Geometry: final body of the model. Coordinates: model frame, mm. Coordinates: 2 decimals unless noted, no trailing zeros. Order: outer loops, then holes, each group sorted by start corner. A loop starts at its lowest first (then second) coordinate and runs counter-clockwise, first axis right, second up. Notation, with made-up numbers: M 27.25,82 L 71.25,82 A17 ccw 71.25,93 Z; hole C 58,64 d8. An arc over 180 degrees is marked long. One line per question, with ' | ' between items.
Autodesk Inventor part; units mm, degrees
ref_plane "YZ Plane" through (0, 0, 0) normal (1, 0, 0) x (0, 1, 0)
ref_plane "XZ Plane" through (0, 0, 0) normal (0, 1, 0) x (-1, 0, 0)
ref_plane "XY Plane" through (0, 0, 0) normal (0, 0, 1) x (1, 0, 0)
sketch "スケッチ1" plane through (0, 0, 0) normal (0, 0, 1) x (1, 0, 0)
  line L0 (51.397, 0) -> (6, 70) construction
  line L1 (51.397, 0) -> (65, -20.9752)
  line L2 (65, -20.9752) -> (25, -44.6993)
  line L3 (0, 0) -> (0, 56.1205) construction
  line L4 (0, 0) -> (51.397, 0) construction
  arc A0 (17.9848, 26.067) -> (17.1698, 21.0636) centre (51.7641, 17.9963) ccw construction
  arc A1 (10.2038, 27.926) -> (9.201, 21.7701) centre (51.7641, 17.9963) ccw construction
  arc A2 (9.201, 21.7701) -> (17.1698, 21.0636) centre (13.1854, 21.4169) ccw construction
  line L5 (13.1854, 21.4169) -> (51.7641, 17.9963) construction
  line L6 (51.7641, 17.9963) -> (13.5604, 24.3596)
  arc A3 (13.5604, 24.3596) -> (13.1854, 21.4169) centre (51.7641, 17.9963) ccw construction
  line L7 (13.1854, 21.4169) -> (66.7927, -23.5971) construction
  line L8 (66.7927, -23.5971) -> (61.9625, 22.6577) construction
  line L9 (13.5604, 24.3596) -> (25, -44.6993)
  line L10 (13.5604, 24.3596) -> (6, 70) construction
  line L11 (13.5604, 24.3596) -> (51.397, 0) construction
  arc A4 (51.397, -25) -> (61.9625, 22.6577) centre (51.397, 0) ccw
  line L12 (25, -44.6993) -> (65, -44.6993) construction
  line L13 (65, -44.6993) -> (65, -20.9752) construction
  line L14 (45, -44.6993) -> (45, -284.6993) construction
  line L15 (51.397, 0) -> (51.9579, -2.4363)
  line L16 (51.397, 0) -> (50.5419, -2.3492) construction
  arc A5 (50.5419, -2.3492) -> (53.1648, 1.7678) centre (51.397, 0) ccw construction
  line L17 (51.397, 0) -> (51.3697, -2.4999) construction
  line L18 (51.397, 0) -> (52.2006, -2.3673) construction
  line L19 (51.397, 0) -> (52.9404, -1.9667) construction
  line L20 (51.397, 0) -> (53.5055, -1.3432) construction
  line L21 (51.397, 0) -> (53.8317, -0.5677) construction
  line L22 (51.397, 0) -> (53.8821, 0.2722) construction
  line L23 (51.397, 0) -> (53.6511, 1.0812) construction
  line L24 (51.397, 0) -> (53.1648, 1.7678) construction
  line L25 (51.7641, 17.9963) -> (51.9579, -2.4363)
  line L26 (50.5419, -2.3492) -> (51.7641, 17.9963) construction
  line L27 (51.7641, 17.9963) -> (53.1648, 1.7678) construction
  line L28 (51.397, -8) -> (51.397, -25) construction
  line L29 (54.051, -7.5469) -> (59.6907, -23.5842) construction
  line L30 (56.4044, -6.2391) -> (67.0451, -19.4971) construction
  line L31 (58.1906, -4.2245) -> (72.6271, -13.2017) construction
  line L32 (59.2074, -1.7315) -> (75.8044, -5.411) construction
  line L33 (59.3395, 0.9576) -> (76.2172, 2.9926) construction
  line L34 (58.572, 3.5383) -> (73.8188, 11.0572) construction
  line L35 (56.9918, 5.7182) -> (68.8808, 17.8694) construction
  line L36 (54.7779, 7.2505) -> (61.9625, 22.6577) construction
  arc A6 (51.397, -8) -> (54.7779, 7.2505) centre (51.397, 0) ccw construction
  line L37 (14.0943, 26.9965) -> (51.7641, 17.9963) construction
  arc A7 (14.0943, 26.9965) -> (13.5604, 24.3596) centre (51.7641, 17.9963) ccw construction
  arc A8 (17.9848, 26.067) -> (10.2038, 27.926) centre (14.0943, 26.9965) ccw construction
  line L38 (51.3697, -2.4999) -> (51.7641, 17.9963) construction
  line L39 (51.7641, 17.9963) -> (13.7589, 25.4541) construction
  line L40 (13.4871, 23.9026) -> (51.7641, 17.9963) construction
  line L41 (52.2006, -2.3673) -> (51.7641, 17.9963) construction
  line L42 (14.0943, 26.9965) -> (8.4208, -42.7732) construction
  line L43 (8.4208, -42.7732) -> (51.397, -25) construction
  line L44 (13.7589, 25.4541) -> (18.1084, -44.4107) construction
  line L45 (18.1084, -44.4107) -> (59.6907, -23.5842) construction
  line L46 (25, -44.6993) -> (45, -284.6993)
  line L47 (65, -20.9752) -> (45, -284.6993)
  line L48 (18.1084, -44.4107) -> (21.0305, -285.2248) construction
  line L49 (21.0305, -285.2248) -> (59.6907, -23.5842) construction
  line L50 (51.397, -25) -> (-6.0328, -283.171) construction
  line L51 (-6.0328, -283.171) -> (8.4208, -42.7732) construction
  line L52 (51.7641, 17.9963) -> (13.2929, 22.4663) construction
  line L53 (51.7641, 17.9963) -> (13.173, 21.2739) construction
  line L54 (51.7641, 17.9963) -> (13.1124, 20.4583) construction
  line L55 (51.7641, 17.9963) -> (13.0939, 20.1483) construction
  line L56 (51.7641, 17.9963) -> (13.1119, 20.4513) construction
  line L57 (51.7641, 17.9963) -> (52.9404, -1.9667) construction
  line L58 (51.7641, 17.9963) -> (53.5055, -1.3432) construction
  line L59 (51.7641, 17.9963) -> (53.8317, -0.5677) construction
  line L60 (51.7641, 17.9963) -> (53.8821, 0.2722) construction
  line L61 (51.7641, 17.9963) -> (53.6511, 1.0812) construction
  line L62 (13.4871, 23.9026) -> (27.8947, -44.5986) construction
  line L63 (27.8947, -44.5986) -> (67.0451, -19.4971) construction
  line L64 (72.6271, -13.2017) -> (37.1961, -43.3261) construction
  line L65 (37.1961, -43.3261) -> (13.2929, 22.4663) construction
  line L66 (13.173, 21.2739) -> (45.5916, -40.7666) construction
  line L67 (45.5916, -40.7666) -> (75.8044, -5.411) construction
  line L68 (76.2172, 2.9926) -> (52.8124, -37.1951) construction
  line L69 (52.8124, -37.1951) -> (13.1124, 20.4583) construction
  line L70 (13.0939, 20.1483) -> (58.7276, -32.9324) construction
  line L71 (58.7276, -32.9324) -> (73.8188, 11.0572) construction
  line L72 (68.8808, 17.8694) -> (63.3391, -28.3055) construction
  line L73 (63.3391, -28.3055) -> (13.1119, 20.4513) construction
  line L74 (27.8947, -44.5986) -> (56.2327, -283.7575) construction
  line L75 (61.9625, 22.6577) -> (293.1766, -105.7574) construction
  line L76 (293.1766, -105.7574) -> (66.7927, -23.5971) construction
  line L77 (68.8808, 17.8694) -> (265.8829, -158.5975) construction
  line L78 (265.8829, -158.5975) -> (63.3391, -28.3055) construction
  line L79 (58.7276, -32.9324) -> (229.4847, -202.7618) construction
  line L80 (229.4847, -202.7618) -> (73.8188, 11.0572) construction
  line L81 (76.2172, 2.9926) -> (187.0489, -237.1465) construction
  line L82 (187.0489, -237.1465) -> (52.8124, -37.1951) construction
  line L83 (45.5916, -40.7666) -> (141.9163, -261.4962) construction
  line L84 (141.9163, -261.4962) -> (75.8044, -5.411) construction
  line L85 (72.6271, -13.2017) -> (97.3466, -276.5254) construction
  line L86 (97.3466, -276.5254) -> (37.1961, -43.3261) construction
  line L87 (56.2327, -283.7575) -> (67.0451, -19.4971) construction
  spline S0 degree 4 poles (-6.0328, -283.171) (-1.0018, -286.6814) (51.7016, -283.757) (37.9506, -286.9352) (110.0397, -275.596) (142.8766, -261.8211) (210.6869, -227.817) (251.1, -183.7947) (281.212, -139.9837) (293.1766, -105.7574) knots 0 0 0 0 0 0.215081 0.31035 0.415619 0.538699 0.666654 1 1 1 1 1 construction
  spline S1 degree 4 poles (8.4208, -42.7732) (14.2837, -44.205) (22.8164, -45.2788) (33.6178, -44.6875) (45.3572, -41.166) (55.0356, -36.4401) (61.2363, -31.2275) (64.7888, -26.7723) (66.7927, -23.5971) knots 0 0 0 0 0 0.340062 0.471566 0.598373 0.71961 1 1 1 1 1
  point P0 (51.397, 0)
  point P1 (51.397, 0)
  point P2 (51.397, 0)
  point P3 (51.397, 0)
  point P4 (51.397, 0)
  point P5 (51.397, 0)
  point P6 (51.397, 0)
  point P7 (51.397, 0)
  dimension "d5" = 70
  dimension "d53" = 45
  dimension "d66" = 25
  dimension "d67" = 40
  dimension "d72" = 240
  dimension "d74" = 20
  dimension "d76" = 2.5
  dimension "d80" = 155
  dimension "d82" = 18
  dimension "d85" = 155
  dimension "d87" = 20
  dimension "d88" = 70
  dimension "d89" = 100
  dimension "d90" = 100
  dimension "d91" = 100
  dimension "d92" = 4
  dimension "d93" = 100
  dimension "d94" = 100
  dimension "d95" = 90
  dimension "d96" = 100
  dimension "d97" = 100
  dimension "d98" = 100
  dimension "d99" = 100
  dimension "d100" = 100
  dimension "d101" = 8
  dimension "d102" = 6
  dimension "d103" = 45
sketch "スケッチ2" plane through (0, 0, 0) normal (0, 0, 1) x (1, 0, 0)
  arc A0 (55.0538, 20.2717) -> (48.4917, 20.2966) centre (51.7641, 17.9963) ccw
  line L0 (40, 3) -> (64, 3) construction
  line L1 (64, 3) -> (64, -9) construction
  line L2 (64, -9) -> (40, -9) construction
  line L3 (40, -9) -> (40, 3) construction
  line L4 (36, 10.1673) -> (36, -48.9437) construction
  line L5 (67, 3) -> (67, -9)
  line L6 (64, -12) -> (40, -12)
  line L7 (37, -9) -> (37, 3)
  arc A1 (37, -9) -> (40, -12) centre (40, -9) ccw
  arc A2 (37.5457, 4.7253) -> (37, 3) centre (40, 3) ccw
  arc A3 (64, -12) -> (67, -9) centre (64, -9) ccw
  line L8 (0, 0) -> (0, -59.5537) construction
  line L9 (10.6628, -3) -> (66.9205, -3) construction
  line L10 (67, 3) -> (55.0538, 20.2717)
  line L11 (37.5457, 4.7253) -> (48.4917, 20.2966)
  dimension "d16" = 24
  dimension "d17" = 4
  dimension "d18" = 12
  dimension "d19" = 3
  dimension "d20" = 72
  dimension "d21" = 3
  dimension "d23" = 4
extrude "押し出し1" add sketch "スケッチ2" along normal blind 2
hole "穴1" at (51.7641, 17.9963, 0) direction (0, 0, 1) diameter 3 end through all
hole "穴2" at (64, 3, 0) at (40, 3, 0) at (40, -9, 0) at (64, -9, 0) direction (0, 0, 1) diameter 2.5 end through all
equation "\"input_link_length\" = 25"
equation "\"input_link_formed_angle\" = 20deg"
equation "\"support_formed_angle\" = 100deg"
equation "\"input_slider_radius\" = 2.5"
equation "\"driver_rotation_range\" = 155deg"
equation "\"virtual_link_length\" = 45"
equation "\"virtual_mass_point_x\" = 6"
equation "\"support_axis_driver_dist\" = 18"
properties part number "COXA_YAW_SERVO_BASE"
1. Section B-B, the plane x = 51. Output: boundary loops of the cut face in (y, z).
Response values:
outline: M -12,0 L 16.71,0 L 16.71,2 L -12,2 Z; M 19.29,0 L 21.92,0 L 21.92,2 L 19.29,2 Z
2. Section C-C, the plane z = 0.7. Output: boundary loops of the cut face in (x, y).
Response values:
outline: M 37,-9 A3 ccw 40,-12 L 64,-12 A3 ccw 67,-9 L 67,3 L 55.05,20.27 A4 ccw 48.49,20.3 L 37.55,4.73 A3 ccw 37,3 Z; hole C 40,-9 d2.5; hole C 40,3 d2.5; hole C 51.76,18 d3; hole C 64,-9 d2.5; hole C 64,3 d2.5
3. Pin query (flat end, axial travel): P1, Ø2, axis at x = 40, y = 3, coming from the +Z side. Return the tip coordinate at first contact, or that it passes through.
Response values:
P1: passes through
4. Section A-A, the plane y = 17. Output: boundary loops of the cut face in (x, z), and give its area (3 significant figures).
Response values:
outline: M 46.17,0 L 50.64,0 L 50.64,2 L 46.17,2 Z; M 52.89,0 L 57.32,0 L 57.32,2 L 52.89,2 Z | area: 17.8 mm^2
5. Draft query along Y for faces 1 (the face through (39.95, -10.25, 1.01)), 2 (the face through (52, -12, 1)), 3 (the face through (52, 1, 2)). Return one class per face: pulls with the +Y half, pulls with the -Y half, needs draft (parallel to the pull), parting line crosses it, or undercut.
Response values:
face 1: undercut | face 2: pulls with the -Y half | face 3: needs draft
6. Material intervals for line 1 (X direction, y = -9, z = 1.25); line 2 (Y direction, x = 40.25, z = 0.6); line 3 (Y direction, x = 40, z = 0.8), sorted ascending. Write a range as [from, to].
Response values:
line 1: x = [37, 38.75], [41.25, 62.75], [65.25, 67] | line 2: y = [-12, -10.22], [-7.78, 1.78], [4.22, 8.57] | line 3: y = [-12, -10.25], [-7.75, 1.75], [4.25, 8.22]
7. Section D-D, the plane x = 43.5. Output: boundary loops of the cut face in (y, z), and give its area (3 significant figures).
Response values:
outline: M -12,0 L 13.2,0 L 13.2,2 L -12,2 Z | area: 50.4 mm^2
